Verification items for the finished model (mm, model axes). A direction names the side the tool comes from. Round coordinates to 2 decimals unless told otherwise and drop trailing zeros. Loops run counter-clockwise (first coordinate to the right, second up) from the corner with the lowest first, then second, coordinate; pieces in that order, holes last. Notation, with made-up numbers: (82, 40.5) -> (107, 40.5) arc R23 ccw to (107, 55.5) -> close; hole circle Ø5 at (55, -12). An arc over 180 degrees is marked (long way). Use a Markdown table: item, result. Add a question column.
```python
from build123d import *

# Parameters (mm, degrees)
SKETCH1_R           = 3
BOSS_EXTRUDE1_DEPTH = 10
FILLET1_R           = 15


with BuildPart() as part:
    # Sketch1 → Boss-Extrude1 (new body)
    with BuildSketch(Plane.XY):
        with BuildLine():
            Line((0, 0), (15, 0))
            Line((15, 0), (15, 10))
            Line((15, 10), (29, 10))
            Line((29, 10), (29, 0))
            Line((29, 0), (44, 0))
            Line((44, 0), (44, 10))
            Line((44, 10), (58, 10))
            Line((58, 10), (58, 0))
            Line((58, 0), (73, 0))
            Line((73, 0), (78.625, -9.742785793))
            Line((78.625, -9.742785793), (83.821152423, -6.742785793))
            Line((83.821152423, -6.742785793), (91.321152423, -19.733166849))
            Line((91.321152423, -19.733166849), (86.125, -22.733166849))
            Line((86.125, -22.733166849), (91.75, -32.475952642))
            Line((91.75, -32.475952642), (96.946152423, -29.475952642))
            Line((96.946152423, -29.475952642), (104.446152423, -42.466333699))
            Line((104.446152423, -42.466333699), (99.25, -45.466333699))
            Line((99.25, -45.466333699), (104.875, -55.209119491))
            Line((104.875, -55.209119491), (110.071152423, -52.209119491))
            Line((110.071152423, -52.209119491), (117.571152423, -65.199500548))
            Line((117.571152423, -65.199500548), (112.375, -68.199500548))
            Line((112.375, -68.199500548), (118, -77.942286341))
            Line((118, -77.942286341), (87.689110868, -95.442286341))
            add(Edge.make_bspline(
                [(87.689110868, -95.442286341), (77.660181341, -75.620017272), (64.817303381, -57.569676854), (49.160476986, -41.291265088)],
                knots=[0, 0, 0, 0, 1, 1, 1, 1], degree=3))
            add(Edge.make_bspline(
                [(0, -25), (17.242534467, -24.639573707), (35.899987596, -27.504326339), (49.160476986, -41.291265088)],
                knots=[0, 0, 0, 0, 1, 1, 1, 1], degree=3))
            Line((0, -25), (0, 0))
        make_face()
        with Locations((23, -18.5)):
            Circle(SKETCH1_R, mode=Mode.SUBTRACT)
    extrude(amount=BOSS_EXTRUDE1_DEPTH)

    # Fillet1
    fillet1_edges = [part.edges().sort_by_distance(p)[0] for p in [
        (87.689110868, -95.442286341, 5),
        (0, -25, 5),
    ]]
    fillet(fillet1_edges, radius=FILLET1_R)


solid = part.part
```
1) Sectioned sample at A-A on x = 107.5. Enter the section's corners in (y, z), then the cut area to 3 significant figures.
2) Release check for a two-part mould opening along Y. For faces 4 (the face through (87.52, -13.15, 4.93)), 5 (the face through (101.88, -43.95, 4.93)), 6 (the face through (15, 5, 5)), 7 (the face through (102.023, -50.27, 4.93)) record: released by +Y, released by -Y, zero draft, split by the parting line, or undercut.
3) Thickness scan on line 1 (X direction, y = 2.5, z = 5.5); line 2 (Y direction, x = 23, z = 3.5); line 3 (X direction, y = -17, z = 9.25). Record the ranges inside material, lowest first.
4) Go/stop test with flat-tipped pins: pin 1 (5 mm diameter, centred on x = 33, z = 5.5, fed in from +Y); pin 2 (1.5 mm diameter, centred on x = 42, z = 4.5, fed in from -Y); pin 3 (5 mm diameter, centred on y = 6, z = 5, fed in from +X). Record where each tip stops, or that it passes through.
5) Access from +Z, -Z, +X, -X, +Y, -Y to the whole of each face (thin tool, end or side, straight path). Record for faces 1 (the face through (113.769, -58.613, 4.93)), 2 (the face through (44, 5, 5)), 3 (the face through (115.01, -66.68, 4.93)).
Geometry results:
| question | item | result |
|---|---|---|
| 1 | outline | (-84, 0) -> (-53.69, 0) -> (-53.69, 10) -> (-84, 10) -> close |
| 1 | area | 303 mm^2 |
| 2 | face 4 | released by +Y |
| 2 | face 5 | undercut |
| 2 | face 6 | zero draft |
| 2 | face 7 | undercut |
| 3 | line 1 | 15 to 29, 44 to 58 |
| 3 | line 2 | -27.05 to -21.5, -15.5 to 10 |
| 3 | line 3 | 1.45 to 20.4, 25.6 to 89.74 |
| 4 | pin 1 | y = 0 |
| 4 | pin 2 | y = -35.72 |
| 4 | pin 3 | x = 58 |
| 5 | face 1 | +Z, -Z, +X, +Y |
| 5 | face 2 | +Z, -Z, +Y |
| 5 | face 3 | +Z, -Z, +X |
